from build123d import *

# Parameters (mm, degrees)
BASE_SKETCH_W                        = 15
BASE_SKETCH_H                        = 15
BASE_SKETCH_EXTRUDE_DEPTH            = 30
CENTER_NUB_CUTOUT_SKETCH_W           = 5
CENTER_NUB_CUTOUT_SKETCH_H           = 15
HINGE_NUB_EXTRUDED_CUT_DEPTH         = 15
HINGE_CUTOUT_SKETCH_W                = 7
HINGE_CUTOUT_SKETCH_H                = 15
HINGE_CUTOUT_EXTRUDED_CUT_DEPTH      = 12
HINGE_HOLE_SKETCH_R                  = 1
HINGE_HOLE_EXTRUDED_CUT_DEPTH        = 35.369317712
CORNER_FILLETS_R                     = 5
STYLE_FILLETS_R                      = 1
ROUTING_HOLES_SKETCH_W               = 2
ROUTING_HOLES_SKETCH_H               = 2
ROUTING_HOLES_EXTRUDED_CUT_DEPTH     = 32.819805153
BACKING_START                        = -3.5
BACKING_EXTRUDE_DEPTH                = 7
EXTRA_ROUTING_CUT_SKETCH_W           = 2
EXTRA_ROUTING_CUT_SKETCH_H           = 10
EXTRA_ROUTING_EXTRUDED_CUT_DEPTH     = 4
ROUTING_FILLETS_R                    = 1
SKETCH2_R                            = 1.75
MIDDLE_SECTION_CONNECTION_HOLE_DEPTH = 3


# Read off the part's stored shape, not the designer's step: Backing Extrude
with BuildPart() as part:
    # Base Sketch → Base Sketch Extrude (new body)
    with BuildSketch(Plane.XY):
        Rectangle(BASE_SKETCH_W, BASE_SKETCH_H)
    extrude(amount=BASE_SKETCH_EXTRUDE_DEPTH)

    # Center Nub Cutout Sketch → Hinge Nub Extruded Cut (cut)
    with BuildSketch(Plane.XY):
        with Locations((5, 0)):
            Rectangle(CENTER_NUB_CUTOUT_SKETCH_W, CENTER_NUB_CUTOUT_SKETCH_H)
        with Locations((-5, 0)):
            Rectangle(CENTER_NUB_CUTOUT_SKETCH_W, CENTER_NUB_CUTOUT_SKETCH_H)
    extrude(amount=HINGE_NUB_EXTRUDED_CUT_DEPTH, mode=Mode.SUBTRACT)

    # Hinge Cutout Sketch → Hinge Cutout Extruded Cut (cut)
    with BuildSketch(Plane.XY.offset(30)):
        Rectangle(HINGE_CUTOUT_SKETCH_W, HINGE_CUTOUT_SKETCH_H)
    extrude(amount=-HINGE_CUTOUT_EXTRUDED_CUT_DEPTH, mode=Mode.SUBTRACT)

    # Hinge Hole Sketch → Hinge Hole Extruded Cut (cut, through all)
    with BuildSketch(Plane(origin=(7.5, 0, 0), x_dir=(0, 0, -1), z_dir=(1, 0, 0))):
        with Locations(Location((-5, 0, 0), (0, 0, 90))):
            Circle(HINGE_HOLE_SKETCH_R)
        with Locations(Location((-27, 0, 0), (0, 0, 90))):
            Circle(HINGE_HOLE_SKETCH_R)
    extrude(amount=-HINGE_HOLE_EXTRUDED_CUT_DEPTH, mode=Mode.SUBTRACT)

    # Corner Fillets
    corner_fillets_edges = [part.edges().sort_by_distance(p)[0] for p in [
        (0, 7.5, 0),
        (-5.5, -7.5, 30),
        (-5.5, 7.5, 30),
        (5.5, -7.5, 30),
        (5.5, 7.5, 30),
    ]]
    fillet(corner_fillets_edges, radius=CORNER_FILLETS_R)

    # Style Fillets
    style_fillets_edges = [part.edges().sort_by_distance(p)[0] for p in [
        (2.5, 7.5, 10),
        (2.5, -7.5, 7.5),
        (7.5, 0, 15),
        (5, 7.5, 15),
        (2.5, 0, 15),
        (5, -7.5, 15),
        (-2.5, -2.5, 0),
        (-2.5, -7.5, 7.5),
        (-2.5, 7.5, 10),
        (-7.5, 0, 15),
        (-5, -7.5, 15),
        (-2.5, 0, 15),
        (-5, 7.5, 15),
        (-7.5, 0, 30),
        (-7.5, -7.5, 20),
        (7.5, -7.5, 20),
        (-7.5, 7.5, 20),
        (-7.5, 6.035533906, 28.535533906),
        (-7.5, -6.035533906, 28.535533906),
        (7.5, 7.5, 20),
        (7.5, 0, 30),
        (7.5, 6.035533906, 28.535533906),
        (7.5, -6.035533906, 28.535533906),
        (-2.5, 6.035533906, 1.464466094),
        (2.5, -2.5, 0),
        (2.5, 6.035533906, 1.464466094),
    ]]
    fillet(style_fillets_edges, radius=STYLE_FILLETS_R)

    # Routing Holes Sketch → Routing Holes Extruded Cut (cut, through all)
    with BuildSketch(Plane.XY):
        with Locations((0, 4.5)):
            Rectangle(ROUTING_HOLES_SKETCH_W, ROUTING_HOLES_SKETCH_H)
        with Locations((0, -4.5)):
            Rectangle(ROUTING_HOLES_SKETCH_W, ROUTING_HOLES_SKETCH_H)
    extrude(amount=ROUTING_HOLES_EXTRUDED_CUT_DEPTH, mode=Mode.SUBTRACT)

    # Backing Extrude outline → Backing Extrude (add)
    with BuildSketch(Plane.YZ.offset(BACKING_START)):
        Polygon((-7.5, 24.05884149), (-7.5, 18), (-5.5, 18), (-5.5, 24.043125728), align=None)
    extrude(amount=BACKING_EXTRUDE_DEPTH)

    # Extra Routing Cut Sketch → Extra Routing Extruded Cut (cut)
    with BuildSketch(Plane(origin=(0, 7.5, 0), x_dir=(1, 0, 0), z_dir=(0, 1, 0))):
        with Locations((0, -6)):
            Rectangle(EXTRA_ROUTING_CUT_SKETCH_W, EXTRA_ROUTING_CUT_SKETCH_H)
    extrude(amount=-EXTRA_ROUTING_EXTRUDED_CUT_DEPTH, mode=Mode.SUBTRACT)

    # Routing Fillets
    routing_fillets_edges = [part.edges().sort_by_distance(p)[0] for p in [
        (-1, -4.5, 18),
        (0, -3.5, 18),
        (1, -4.5, 18),
        (-1, 4.5, 18),
        (0, 3.5, 18),
        (1, 4.5, 18),
        (0, 5.5, 18),
        (0, -5.5, 0),
        (0, -3.5, 0),
        (0, 5.5, 11),
    ]]
    fillet(routing_fillets_edges, radius=ROUTING_FILLETS_R)

    # Sketch2 → Middle Section Connection Hole (cut)
    with BuildSketch(Plane(origin=(7.5, 0, 0), x_dir=(0, 0, -1), z_dir=(1, 0, 0))):
        with Locations(Location((-21, 0, 0), (0, 0, 90))):
            Circle(SKETCH2_R)
    middle_section_connection_hole = extrude(amount=-MIDDLE_SECTION_CONNECTION_HOLE_DEPTH, mode=Mode.SUBTRACT)

    # Mirror1: Middle Section Connection Hole across plane
    add(middle_section_connection_hole.mirror(Plane(origin=(0, 0, 0), x_dir=(0, 0, 1), z_dir=(1, 0, 0))), mode=Mode.SUBTRACT)


solid = part.part
Part model, mm, in its own coordinate system. A direction names the side the tool comes from. Coordinates: 2 decimals unless noted, no trailing zeros. Loops run counter-clockwise (first coordinate to the right, second up) from the corner with the lowest first, then second, coordinate; pieces in that order, holes last. Notation, with made-up numbers: (43.25, 69.5) -> (52.25, 69.5) arc R16 cw to (52.25, 89.5) -> close; hole circle Ø8 at (-6.5, 36.5). An arc over 180 degrees is marked (long way). Use a Markdown table: item, result. Add a question column.
Item 1: Band-saw the part on A-A on x = 0. Write the cut outline in (y, z).
Item 2: Probe probe 1 along Z at (x, y) = (6.6, 0); probe 2 along Z at (x, y) = (4.75, -0.75); probe 3 along X at (y, z) = (-1.25, 24). List the from-to ranges inside material, lowest first.
Item 3: Pull direction Z, two halves, no side cores. Call faces 1 (the cylindrical face through (6.021, -0.228, 22.735)), 2 (the flat face through (0, 1, 18)), 3 (the flat face through (-1, 7.5, 16)): +Z half, -Z half, draft (parallel to the pull), parting line (faces both ways), or undercut.
Item 4: Which spindle directions (+Z, -Z, +X, -X, +Y, -Y) get a long thin tool onto all of the face, cutting with end or side? Do faces 4 (the flat face through (0, -5.5, 15)), 5 (the flat face through (4.5, 0, 21)), 6 (the flat face through (0, 7, 11)), 7 (the cylindrical face through (-4.979, 7.199, 15.285)), 8 (the cylindrical face through (5.021, 7.215, 15.301)). Say none if no direction does.
Item 5: Flat gauge pins, fed straight in: P1, Ø1.5, axis at y = -0.5, z = 11.5, coming from the +X side; P2, Ø4, axis at x = 0, z = 25, coming from the +Y side; P3, Ø1.2, axis at y = 5.5, z = 6, coming from the -X side. Where does each tip first touch, or does it go through?
Item 6: Band-saw the part on B-B on z = 10.5. Write the cut outline in (x, y), plus the area to 3 significant figures.
Item 7: Band-saw the part on D-D on z = 21. Write the cut outline in (x, y).
Item 8: Band-saw the part on C-C on x = -4. Write the cut outline in (y, z), plus the area to 3 significant figures.
Geometry says:
| question | item | result |
|---|---|---|
| 1 | outline | (-7.5, 0) -> (-6.5, 0) arc R1 ccw to (-5.5, 1) -> (-5.5, 24.04) -> (-7.5, 24.06) -> close; (-3.5, 1) arc R1 ccw to (-2.5, 0) -> (2.5, 0) arc R5 ccw to (3.5, 0.1) -> (3.5, 17) arc R1 ccw to (2.5, 18) -> (-2.5, 18) arc R1 ccw to (-3.5, 17) -> close; (5.5, 12) arc R1 ccw to (6.5, 11) -> (7.5, 11) -> (7.5, 18) -> (6.5, 18) arc R1 ccw to (5.5, 17) -> close; hole circle Ø2 at (0, 5) |
| 2 | probe 1 | 15.01 to 19.25, 22.75 to 26, 28 to 29.99 |
| 2 | probe 2 | 15 to 19.42, 22.58 to 26.34, 27.66 to 30 |
| 2 | probe 3 | -7.5 to -3.5, 3.5 to 7.5 |
| 3 | face 1 | undercut |
| 3 | face 2 | +Z half |
| 3 | face 3 | draft |
| 4 | face 4 | +Z |
| 4 | face 5 | +X |
| 4 | face 6 | -Z, +Y |
| 4 | face 7 | -Z, -X, +Y |
| 4 | face 8 | -Z, +X, +Y |
| 5 | P1 | x = 2.5 |
| 5 | P2 | y = -5.5 |
| 5 | P3 | x = -2.5 |
| 6 | outline | (-2.5, -6.5) arc R1 ccw to (-1.5, -7.5) -> (1.5, -7.5) arc R1 ccw to (2.5, -6.5) -> (2.5, 6.5) arc R1 ccw to (1.5, 7.5) -> (1, 7.5) -> (1, 3.5) -> (-1, 3.5) -> (-1, 7.5) -> (-1.5, 7.5) arc R1 ccw to (-2.5, 6.5) -> close; hole (-1, -5.5) -> (1, -5.5) -> (1, -3.5) -> (-1, -3.5) -> close |
| 6 | area | 62.1 mm² |
| 7 | outline | (-7.5, -6.5) arc R1 ccw to (-6.5, -7.5) -> (6.5, -7.5) arc R1 ccw to (7.5, -6.5) -> (7.5, -1.75) -> (4.5, -1.75) -> (4.5, 1.75) -> (7.5, 1.75) -> (7.5, 6.5) arc R1 ccw to (6.5, 7.5) -> (3.5, 7.5) -> (3.5, -5.5) -> (-3.5, -5.5) -> (-3.5, 7.5) -> (-6.5, 7.5) arc R1 ccw to (-7.5, 6.5) -> (-7.5, 1.75) -> (-4.5, 1.75) -> (-4.5, -1.75) -> (-7.5, -1.75) -> close |
| 8 | outline | (-7.5, 16) arc R1 ccw to (-6.5, 15) -> (6.5, 15) arc R1 ccw to (7.5, 16) -> (7.5, 25) arc R5 ccw to (2.5, 30) -> (-2.5, 30) arc R5 ccw to (-7.5, 25) -> close; hole circle Ø2 at (0, 27) |
| 8 | area | 211 mm² |
